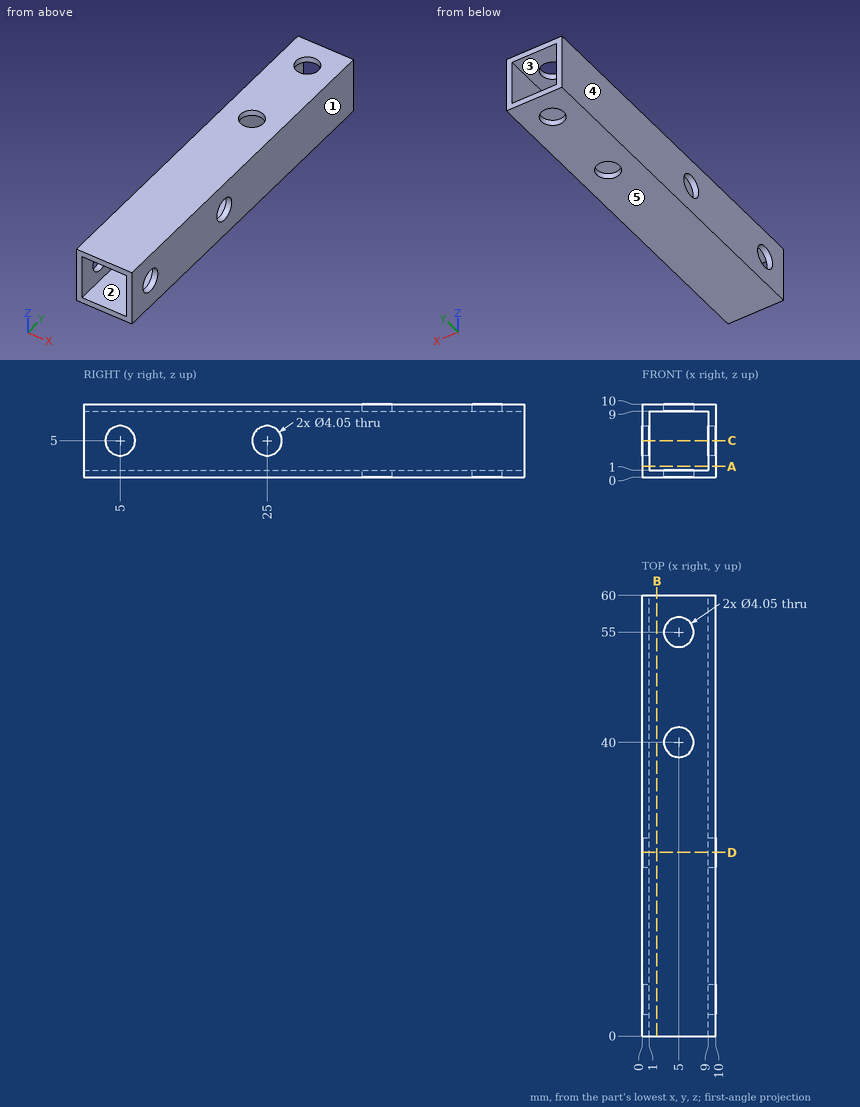
Part print with two shaded views. Sizes in mm from the minimum x, y, z corner. A direction names the side the tool comes from. Round coordinates to 2 decimals unless told otherwise and drop trailing zeros. Loops run counter-clockwise (first coordinate to the right, second up) from the corner with the lowest first, then second, coordinate; pieces in that order, holes last.
Item 1: Two-plate mould, pull along Z, no slides. Class the marked faces 3, 4 and 5: released by +Z, released by -Z, zero draft, split by the parting line, or undercut.
Item 2: Which spindle directions (+Z, -Z, +X, -X, +Y, -Y) get a long thin tool onto all of the face, cutting with end or side? Do the marked faces 1 and 2. Say none if no direction does.
Item 3: Saw through at A-A (z = 1.5). List the corners of the cut face in (x, y), then the cut area to 3 significant figures.
Item 4: Saw through at B-B (x = 2). List the corners of the cut face in (y, z), then the cut area to 3 significant figures.
Item 5: Pin check, flat tip, straight feed: P1, Ø6, axis at x = 7.5, z = 1, coming from the -Y side. Stop position of the tip, or through.
Item 6: Saw through at D-D (y = 25). List the corners of the cut face in (x, z) (3 decimals), then the cut area to 3 significant figures.
Item 7: Saw through at C-C (z = 5). List the corners of the cut face in (x, y) (3 decimals).
Item 8: Drill centre lines: line 1 along Y through (x, z) = (0.4, 5) (3 decimals); line 2 along Y through (x, z) = (5, 9.45) (3 decimals); line 3 along X through (y, z) = (5, 7.25). Where is each one in solid material? Low to high.
Worked answers:
1. face 3: undercut
1. face 4: zero draft
1. face 5: released by -Z
2. face 1: +Z, -Z, +X, +Y, -Y
2. face 2: +Y, -Y
3. outline: (0, 0) - (1, 0) - (1, 60) - (0, 60) - close; (9, 0) - (10, 0) - (10, 60) - (9, 60) - close
3. area: 120 mm2
4. outline: (0, 0) - (60, 0) - (60, 1) - (0, 1) - close; (0, 9) - (60, 9) - (60, 10) - (0, 10) - close
4. area: 120 mm2
5. P1: stops at y = 0
6. outline: (0, 0) - (10, 0) - (10, 2.975) - (9, 2.975) - (9, 1) - (1, 1) - (1, 2.975) - (0, 2.975) - close; (0, 7.025) - (1, 7.025) - (1, 9) - (9, 9) - (9, 7.025) - (10, 7.025) - (10, 10) - (0, 10) - close
6. area: 27.9 mm2
7. outline: (0, 0) - (1, 0) - (1, 2.975) - (0, 2.975) - close; (0, 7.025) - (1, 7.025) - (1, 22.975) - (0, 22.975) - close; (0, 27.025) - (1, 27.025) - (1, 60) - (0, 60) - close; (9, 0) - (10, 0) - (10, 2.975) - (9, 2.975) - close; (9, 7.025) - (10, 7.025) - (10, 22.975) - (9, 22.975) - close; (9, 27.025) - (10, 27.025) - (10, 60) - (9, 60) - close
8. line 1: y = 0 to 2.975, 7.025 to 22.975, 27.025 to 60
8. line 2: y = 0 to 37.975, 42.025 to 52.975, 57.025 to 60
8. line 3: x = 0 to 1, 9 to 10
